Can you work these out from the model? Positions are in its coordinate system, mm. A direction names the side the tool comes from. Round coordinates to 2 decimals unless told otherwise and drop trailing zeros. Loops run counter-clockwise (first coordinate to the right, second up) from the corner with the lowest first, then second, coordinate; pieces in that order, holes last. Notation, with made-up numbers: (58, -14) -> (104, -14) arc R29 cw to (104, 24) -> close; hole circle Ø7 at (42.5, 64.25). An arc over 180 degrees is marked (long way). Use a Markdown table: item, result.
from build123d import *

# Parameters (mm, degrees)
SKETCH_1_R          = 1.075
SKETCH_1_R_2        = 1.55
SKETCH_1_R_3        = 3.15
SKETCH_1_R_4        = 3.150000003
EXTRUDE_1_DEPTH     = 2.5
CUT_EXTRUDE_1_REACH = 97.864
FILLET_1_R          = 3
CUT_EXTRUDE_2_REACH = 97.864
SKETCH_4_W          = 3.5
SKETCH_4_H          = 6.5


with BuildPart() as part:
    # 草图1 → 凸台-拉伸1 (new body)
    with BuildSketch(Plane(origin=(0, 0, 0), x_dir=(1, 0, 0), z_dir=(0, 1, 0))):
        with BuildLine():
            Line((74.268493783, -46.542811359), (63.739297222, -38.892902272))
            ThreePointArc((63.739297222, -38.892902272), (43.92237371, 0), (63.739297222, 38.892902272))
            Line((63.739297222, 38.892902272), (74.268493783, 46.542811359))
            ThreePointArc((74.268493783, 46.542811359), (75.595884236, 54.923624839), (67.215070756, 56.251015292))
            Line((67.215070756, 56.251015292), (56.685874194, 48.601106204))
            ThreePointArc((56.685874194, 48.601106204), (0, 33.998472353), (-56.685874194, 48.601106204))
            Line((-56.685874194, 48.601106204), (-67.215070756, 56.251015292))
            ThreePointArc((-67.215070756, 56.251015292), (-75.595884236, 54.923624839), (-74.268493783, 46.542811359))
            Line((-74.268493783, 46.542811359), (-63.739297222, 38.892902272))
            ThreePointArc((-63.739297222, 38.892902272), (-43.92237371, 0), (-63.739297222, -38.892902272))
            Line((-63.739297222, -38.892902272), (-74.268493783, -46.542811359))
            ThreePointArc((-74.268493783, -46.542811359), (-75.595884236, -54.923624839), (-67.215070756, -56.251015292))
            Line((-67.215070756, -56.251015292), (-56.685874194, -48.601106204))
            ThreePointArc((-56.685874194, -48.601106204), (0, -33.998472353), (56.685874194, -48.601106204))
            Line((56.685874194, -48.601106204), (67.215070756, -56.251015292))
            ThreePointArc((67.215070756, -56.251015292), (75.595884236, -54.923624839), (74.268493783, -46.542811359))
        make_face()
        with Locations(Location((10, 10, 0), (0, 0, 270))):
            Circle(SKETCH_1_R, mode=Mode.SUBTRACT)
        with Locations(Location((12.75, 12.75, 0), (0, 0, 270))):
            Circle(SKETCH_1_R, mode=Mode.SUBTRACT)
        with Locations(Location((15.25, 15.25, 0), (0, 0, 270))):
            Circle(SKETCH_1_R_2, mode=Mode.SUBTRACT)
        with Locations(Location((15.25, -15.25, 0), (0, 0, 90))):
            Circle(SKETCH_1_R_2, mode=Mode.SUBTRACT)
        with Locations(Location((12.75, -12.75, 0), (0, 0, 90))):
            Circle(SKETCH_1_R, mode=Mode.SUBTRACT)
        with Locations(Location((10, -10, 0), (0, 0, 90))):
            Circle(SKETCH_1_R, mode=Mode.SUBTRACT)
        with Locations(Location((28, -28, 0), (0, 0, 90))):
            Circle(SKETCH_1_R_3, mode=Mode.SUBTRACT)
        with Locations(Location((28, 28, 0), (0, 0, 270))):
            Circle(SKETCH_1_R_4, mode=Mode.SUBTRACT)
        with Locations(Location((44.044221455, -32, 0), (0, 0, 270))):
            Circle(SKETCH_1_R_2, mode=Mode.SUBTRACT)
        with Locations(Location((60.224561343, -43.755705046, 0), (0, 0, 270))):
            Circle(SKETCH_1_R_2, mode=Mode.SUBTRACT)
        with Locations(Location((60.224561343, 43.755705046, 0), (0, 0, 90))):
            Circle(SKETCH_1_R_2, mode=Mode.SUBTRACT)
        with Locations(Location((44.044221455, 32, 0), (0, 0, 90))):
            Circle(SKETCH_1_R_2, mode=Mode.SUBTRACT)
        with Locations(Location((-44.044221455, 32, 0), (0, 0, 270))):
            Circle(SKETCH_1_R_2, mode=Mode.SUBTRACT)
        with Locations(Location((-60.224561343, 43.755705046, 0), (0, 0, 270))):
            Circle(SKETCH_1_R_2, mode=Mode.SUBTRACT)
        with Locations(Location((-60.224561343, -43.755705046, 0), (0, 0, 90))):
            Circle(SKETCH_1_R_2, mode=Mode.SUBTRACT)
        with Locations(Location((-44.044221455, -32, 0), (0, 0, 90))):
            Circle(SKETCH_1_R_2, mode=Mode.SUBTRACT)
        with Locations(Location((-28, 28, 0), (0, 0, 90))):
            Circle(SKETCH_1_R_4, mode=Mode.SUBTRACT)
        with Locations(Location((-28, -28, 0), (0, 0, 270))):
            Circle(SKETCH_1_R_3, mode=Mode.SUBTRACT)
        with Locations(Location((-10, -10, 0), (0, 0, 270))):
            Circle(SKETCH_1_R, mode=Mode.SUBTRACT)
        with Locations(Location((-12.75, -12.75, 0), (0, 0, 270))):
            Circle(SKETCH_1_R, mode=Mode.SUBTRACT)
        with Locations(Location((-15.25, -15.25, 0), (0, 0, 270))):
            Circle(SKETCH_1_R_2, mode=Mode.SUBTRACT)
        with Locations(Location((-15.25, 15.25, 0), (0, 0, 90))):
            Circle(SKETCH_1_R_2, mode=Mode.SUBTRACT)
        with Locations(Location((-12.75, 12.75, 0), (0, 0, 90))):
            Circle(SKETCH_1_R, mode=Mode.SUBTRACT)
        with Locations(Location((-10, 10, 0), (0, 0, 90))):
            Circle(SKETCH_1_R, mode=Mode.SUBTRACT)
    extrude(amount=EXTRUDE_1_DEPTH)

    # 草图2 → 切除-拉伸1 (cut, up to next)
    with BuildSketch(Plane(origin=(0, 2.5, 0), x_dir=(1, 0, 0), z_dir=(0, 1, 0)), mode=Mode.PRIVATE) as cut_extrude_1_sk1:
        with BuildLine():
            Line((-23.801448899, 14.429581723), (-9.371867176, 0))
            Line((-9.371867176, 0), (-23.801448899, -14.429581723))
            ThreePointArc((-23.801448899, -14.429581723), (-26.692624222, -17.058284994), (-29.820182402, -19.400795498))
            ThreePointArc((-29.820182402, -19.400795498), (-26.863678166, 0), (-29.820182402, 19.400795498))
            ThreePointArc((-29.820182402, 19.400795498), (-26.692624222, 17.058284994), (-23.801448899, 14.429581723))
        make_face()
    cut_extrude_1_tool1 = extrude(cut_extrude_1_sk1.sketch, amount=-CUT_EXTRUDE_1_REACH, mode=Mode.PRIVATE) & part.part
    # 草图2 → 切除-拉伸1 (cut, up to next)
    with BuildSketch(Plane(origin=(0, 2.5, 0), x_dir=(1, 0, 0), z_dir=(0, 1, 0)), mode=Mode.PRIVATE) as cut_extrude_1_sk2:
        with BuildLine():
            Line((14.429581723, 23.801448899), (0, 9.371867176))
            Line((0, 9.371867176), (-14.429581723, 23.801448899))
            ThreePointArc((-14.429581723, 23.801448899), (-17.058284994, 26.692624222), (-19.400795498, 29.820182402))
            ThreePointArc((-19.400795498, 29.820182402), (0, 26.863678166), (19.400795498, 29.820182402))
            ThreePointArc((19.400795498, 29.820182402), (17.058284994, 26.692624222), (14.429581723, 23.801448899))
        make_face()
    cut_extrude_1_tool2 = extrude(cut_extrude_1_sk2.sketch, amount=-CUT_EXTRUDE_1_REACH, mode=Mode.PRIVATE) & part.part
    # 草图2 → 切除-拉伸1 (cut, up to next)
    with BuildSketch(Plane(origin=(0, 2.5, 0), x_dir=(1, 0, 0), z_dir=(0, 1, 0)), mode=Mode.PRIVATE) as cut_extrude_1_sk3:
        with BuildLine():
            Line((23.801448899, -14.429581723), (9.371867176, 0))
            Line((9.371867176, 0), (23.801448899, 14.429581723))
            ThreePointArc((23.801448899, 14.429581723), (26.692624222, 17.058284994), (29.820182402, 19.400795498))
            ThreePointArc((29.820182402, 19.400795498), (26.863678166, 0), (29.820182402, -19.400795498))
            ThreePointArc((29.820182402, -19.400795498), (26.692624222, -17.058284994), (23.801448899, -14.429581723))
        make_face()
    cut_extrude_1_tool3 = extrude(cut_extrude_1_sk3.sketch, amount=-CUT_EXTRUDE_1_REACH, mode=Mode.PRIVATE) & part.part
    # 草图2 → 切除-拉伸1 (cut, up to next)
    with BuildSketch(Plane(origin=(0, 2.5, 0), x_dir=(1, 0, 0), z_dir=(0, 1, 0)), mode=Mode.PRIVATE) as cut_extrude_1_sk4:
        with BuildLine():
            Line((-14.429581723, -23.801448899), (0, -9.371867176))
            Line((0, -9.371867176), (14.429581723, -23.801448899))
            ThreePointArc((14.429581723, -23.801448899), (17.058284994, -26.692624222), (19.400795498, -29.820182402))
            ThreePointArc((19.400795498, -29.820182402), (0, -26.863678166), (-19.400795498, -29.820182402))
            ThreePointArc((-19.400795498, -29.820182402), (-17.058284994, -26.692624222), (-14.429581723, -23.801448899))
        make_face()
    cut_extrude_1_tool4 = extrude(cut_extrude_1_sk4.sketch, amount=-CUT_EXTRUDE_1_REACH, mode=Mode.PRIVATE) & part.part
    add(cut_extrude_1_tool1.solids().sort_by_distance((-21.651527, 2.5, 0))[0], mode=Mode.SUBTRACT)
    add(cut_extrude_1_tool2.solids().sort_by_distance((0, 2.5, -21.651527))[0], mode=Mode.SUBTRACT)
    add(cut_extrude_1_tool3.solids().sort_by_distance((21.651527, 2.5, 0))[0], mode=Mode.SUBTRACT)
    add(cut_extrude_1_tool4.solids().sort_by_distance((0, 2.5, 21.651527))[0], mode=Mode.SUBTRACT)

    # 圆角1
    fillet_1_edges = [part.edges().sort_by_distance(p)[0] for p in [
        (9.371867176, 1.25, 0),
        (0, 1.25, -9.371867176),
        (0, 1.25, 9.371867176),
        (-9.371867176, 1.25, 0),
    ]]
    fillet(fillet_1_edges, radius=FILLET_1_R)

    # 草图4 → 切除-拉伸2 (cut, up to next)
    with BuildSketch(Plane(origin=(0, 2.5, 0), x_dir=(1, 0, 0), z_dir=(0, 1, 0)), mode=Mode.PRIVATE) as cut_extrude_2_sk1:
        with Locations((34.75, 0)):
            Rectangle(SKETCH_4_W, SKETCH_4_H)
    cut_extrude_2_tool1 = extrude(cut_extrude_2_sk1.sketch, amount=-CUT_EXTRUDE_2_REACH, mode=Mode.PRIVATE) & part.part
    # 草图4 → 切除-拉伸2 (cut, up to next)
    with BuildSketch(Plane(origin=(0, 2.5, 0), x_dir=(1, 0, 0), z_dir=(0, 1, 0)), mode=Mode.PRIVATE) as cut_extrude_2_sk2:
        with Locations((-34.75, 0)):
            Rectangle(SKETCH_4_W, SKETCH_4_H)
    cut_extrude_2_tool2 = extrude(cut_extrude_2_sk2.sketch, amount=-CUT_EXTRUDE_2_REACH, mode=Mode.PRIVATE) & part.part
    add(cut_extrude_2_tool1.solids().sort_by_distance((34.75, 2.5, 0))[0], mode=Mode.SUBTRACT)
    add(cut_extrude_2_tool2.solids().sort_by_distance((-34.75, 2.5, 0))[0], mode=Mode.SUBTRACT)


solid = part.part
1. I want a section at A-A (x = 0). Please give me the cut outline in (y, z), plus the area to 3 significant figures.
Answer sheet:
| item | result |
|---|---|
| outline | (0, -34) -> (2.5, -34) -> (2.5, -26.86) -> (0, -26.86) -> close; (0, -10.61) -> (2.5, -10.61) -> (2.5, 10.61) -> (0, 10.61) -> close; (0, 26.86) -> (2.5, 26.86) -> (2.5, 34) -> (0, 34) -> close |
| area | 88.7 mm² |
2. If we mould it in two halves opening along Z, with no side actions, what happens to faces 1 (the cylindrical face through (-61.6, 1.23, -43.04)), 2 (the flat face through (0, 0, -5)), 3 (the flat face through (-62.024, 1.232, 52.48))? For each: +Z half, -Z half, draft (parallel to the pull), parting line (faces both ways), or undercut.
Answer sheet:
| item | result |
|---|---|
| face 1 | undercut |
| face 2 | draft |
| face 3 | +Z half |
3. Will these pins go through, and if not, where does the flat tip stop? pin 1 Ø1.7 at (x, z) = (12.75, 12.75) entering from +Y; pin 2 Ø1.5 at (y, z) = (0.5, -31.5) entering from +X; pin 3 Ø0.8 at (x, y) = (-34.5, 2) entering from +Z; pin 4 Ø1.2 at (x, y) = (35, 1.5) entering from +Z.
Answer sheet:
| item | result |
|---|---|
| pin 1 | passes through |
| pin 2 | stops at x = 56.34 |
| pin 3 | stops at z = 39.31 |
| pin 4 | stops at z = 39.53 |
4. Which directions (+Z, -Z, +X, -X, +Y, -Y) give clear straight access to the entire face, cutting with the end or side of a thin tool? Please do faces 4 (the flat face through (-69.078, 1.232, -42.771)), 5 (the flat face through (61.877, 1.232, 52.373)), 6 (the flat face through (-8.36, 1.27, 17.73)), 7 (the flat face through (68.93, 1.232, -42.664)).
Answer sheet:
| item | result |
|---|---|
| face 4 | -X, +Y, -Y |
| face 5 | +Z, +Y, -Y |
| face 6 | +Y, -Y |
| face 7 | +X, +Y, -Y |
5. I want a section at C-C (y = 0.9). State how many separate pieces and enclosed holes the cut face has, plus the area to 3 significant figures.
Answer sheet:
| item | result |
|---|---|
| separate pieces | 1 |
| enclosed holes | 30 |
| area | 7,080 mm² |
6. I need wall thicknesses on line 1 (X direction, y = 1.3, z = -15.25); line 2 (X direction, y = 2, z = -5.5); line 3 (X direction, y = 1.65, z = -12.75) (3 decimals). Which ranges of each line are inside material? Lowest first, please.
Answer sheet:
| item | result |
|---|---|
| line 1 | x = -46.41 to -28.67, -24.65 to -16.8, -13.7 to -5.88, 5.88 to 13.7, 16.8 to 24.65, 28.67 to 46.41 |
| line 2 | x = -44.24 to -27.1, -14.87 to 14.87, 27.1 to 44.24 |
| line 3 | x = -45.644 to -28.124, -22.122 to -13.825, -11.675 to -3.378, 3.378 to 11.675, 13.825 to 22.122, 28.124 to 45.644 |
7. I want a section at B-B (z = -36). Please give me the cut outline in (x, y), plus the area to 3 significant figures.
Answer sheet:
| item | result |
|---|---|
| outline | (-60.14, 0) -> (-21.58, 0) -> (-21.58, 2.5) -> (-60.14, 2.5) -> close; (21.58, 0) -> (60.14, 0) -> (60.14, 2.5) -> (21.58, 2.5) -> close |
| area | 193 mm² |
